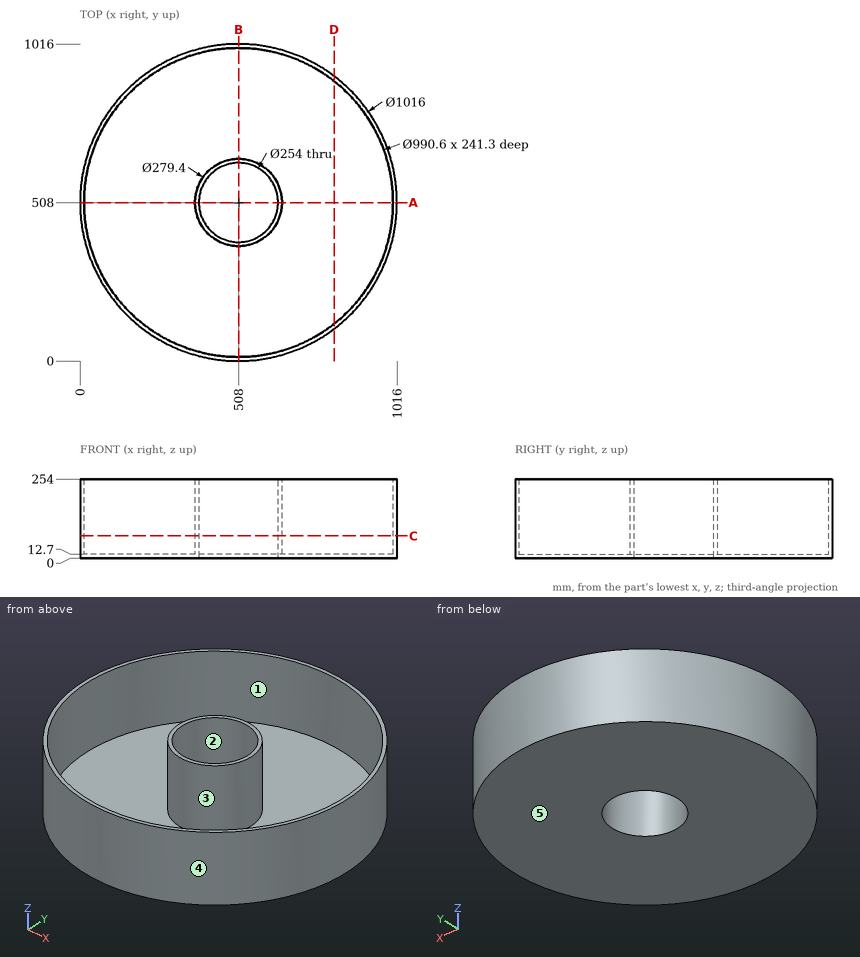
Input: dimensioned drawing with shaded views. Units: mm. Origin: part minimum x, y, z. A direction names the side the tool comes from. Give positions to 0.01 mm unless a question says otherwise; leave off trailing zeros. Write each loop counter-clockwise with the first axis right and the second up, starting at its lowest first coordinate (ties: lowest second). Pieces come first, ordered by that corner, then holes. Notation, with made-up numbers: (29, 15.5) -> (83, 15.5) arc R10 ccw to (83, 27.5) -> close; hole circle Ø7 at (50, 8). An arc over 180 degrees is marked (long way). Return JSON: item names as keys, results as strings. Group by question number.
1. Section C-C, the plane z = 71.5. Output: boundary loops of the cut face in (x, y).
2. Mould query, pull axis X, two halves, no side actions, for the marked faces 3, 4 and 5. Classes: +X half, -X half, draft (parallel to the pull), parting line (faces both ways), or undercut.
3. Section A-A, the plane y = 508. Output: boundary loops of the cut face in (x, z), then the cut area to 3 significant figures.
4. Pin query (flat end, axial travel): pin 1 Ø1.5 at (y, z) = (652.5, 103) entering from +X; pin 2 Ø5 at (x, z) = (244.5, 216) entering from +Y; pin 3 Ø12 at (x, y) = (660, 333.5) entering from +Z. Return the tip coordinate at first contact, or that it passes through.
5. Material intervals for line 1 (Y direction, x = 508, z = 91); line 2 (Y direction, x = 406, z = 68); line 3 (Z direction, x = 452.5, y = 171.5), sorted ascending. Write a range as from..to.
6. Access query for the marked faces 1 and 2. Directions: +Z, -Z, +X, -X, +Y, -Y. A direction counts if a zero-diameter tool reaches every point of the face in a straight line with its end or side. Return the directions, or none.
7. Section D-D, the plane x = 814.5. Output: boundary loops of the cut face in (y, z).
Determined:
{
 "1": {"outline": "circle Ø1016 at (508, 508); circle Ø279.4 at (508, 508); hole circle Ø990.6 at (508, 508); hole circle Ø254 at (508, 508)"},
 "2": {"face 3": "undercut", "face 4": "parting line", "face 5": "draft"},
 "3": {"outline": "(0, 0) -> (381, 0) -> (381, 254) -> (368.3, 254) -> (368.3, 12.7) -> (12.7, 12.7) -> (12.7, 254) -> (0, 254) -> close; (635, 0) -> (1016, 0) -> (1016, 254) -> (1003.3, 254) -> (1003.3, 12.7) -> (647.7, 12.7) -> (647.7, 254) -> (635, 254) -> close", "area": "21,900 mm2"},
 "4": {"pin 1": "stops at x = 995.24", "pin 2": "stops at y = 943.82", "pin 3": "stops at z = 12.7"},
 "5": {"line 1": "y = 0..12.7, 368.3..381, 635..647.7, 1003.3..1016", "line 2": "y = 10.35..23.32, 412.54..432.34, 583.66..603.46, 992.68..1005.65", "line 3": "z = 0..12.7"},
 "6": {"face 1": "+Z", "face 2": "+Z, -Z"},
 "7": {"outline": "(102.88, 0) -> (913.12, 0) -> (913.12, 254) -> (897.08, 254) -> (897.08, 12.7) -> (118.92, 12.7) -> (118.92, 254) -> (102.88, 254) -> close"}
}
